Geometry check sheet. Reference: the model listing, model coordinates, mm. Face numbers are marked on the shaded views. A direction names the side the tool comes from. Give positions to 0.01 mm unless a question says otherwise; leave off trailing zeros. Loops run counter-clockwise (first coordinate to the right, second up) from the corner with the lowest first, then second, coordinate; pieces in that order, holes last. Notation, with made-up numbers: (84.25, 15) -> (143.25, 15) arc R16 ccw to (143.25, 44) -> close; hole circle Ø9 at (18.25, -29.75). An arc over 180 degrees is marked (long way). Write item = value, one per line.
```python
from build123d import *

# Parameters (mm, degrees)
ENLEV_MAT_EXTRU_1_DEPTH = 1.2
ESQUISSE3_W             = 2.5
ESQUISSE3_H             = 6
CHANFREIN1_SIZE         = 0.5
ENL_V_MAT_EXTRU_1_DEPTH = 2


with BuildPart() as part:
    # Esquisse1 → Base-R_volution (revolve)
    with BuildSketch(Plane(origin=(0, 0, 0), x_dir=(1, 0, 0), z_dir=(0, 1, 0)), mode=Mode.PRIVATE) as base_r_volution_sk:
        with BuildLine():
            Line((0, 0), (3.85, 0))
            Line((3.85, 0), (3.85, 1.47314887))
            ThreePointArc((3.85, 1.47314887), (3.806875399, 1.689977873), (3.684065354, 1.873804531))
            ThreePointArc((3.684065354, 1.873804531), (1.993841151, 3.003350962), (0, 3.4))
            Line((0, 3.4), (0, 0))
        make_face()
    revolve(base_r_volution_sk.sketch.rotate(Axis((0, 0, 0), (0, 0, -1)), 180), axis=Axis((0, 0, 0), (0, 0, -1)))

    # Esquisse2 → Enlev. mat.-Extru.1 (cut)
    with BuildSketch(Plane.XY.offset(-3.4)):
        Polygon((0.6, -0.6), (0.6, -2.35), (-0.6, -2.35), (-0.6, -0.6), (-2.35, -0.6), (-2.35, 0.6), (-0.6, 0.6), (-0.6, 2.35), (0.6, 2.35), (0.6, 0.6), (2.35, 0.6), (2.35, -0.6), align=None)
    extrude(amount=ENLEV_MAT_EXTRU_1_DEPTH, mode=Mode.SUBTRACT)

    # Esquisse3 → Boss.-R_vol.1 (revolve)
    with BuildSketch(Plane(origin=(0, 0, 0), x_dir=(1, 0, 0), z_dir=(0, 1, 0)), mode=Mode.PRIVATE) as boss_r_vol_1_sk:
        with Locations((1.25, -3)):
            Rectangle(ESQUISSE3_W, ESQUISSE3_H)
    revolve(boss_r_vol_1_sk.sketch.rotate(Axis((0, 0, 0), (0, 0, 1)), 345.677280022), axis=Axis((0, 0, 0), (0, 0, 1)))

    # Chanfrein1
    chanfrein1_edges = [part.edges().sort_by_distance(p)[0] for p in [
        (-2.422294277, 0.618458113, 6),
    ]]
    chamfer(chanfrein1_edges, length=CHANFREIN1_SIZE)

    # Esquisse6 → Enl_v. mat.-Extru.1 (cut)
    with BuildSketch(Plane(origin=(0, 0, -2.2), x_dir=(-1, 0, 0), z_dir=(0, 0, -1))):
        Polygon((2.35, -0.6), (2.35, 0.6), (0.6, 0.6), (0.6, 2.35), (-0.6, 2.35), (-0.6, 0.6), (-2.35, 0.6), (-2.35, -0.6), (-0.6, -0.6), (-0.6, -2.35), (0.6, -2.35), (0.6, -0.6), align=None)
    extrude(amount=-ENL_V_MAT_EXTRU_1_DEPTH, mode=Mode.SUBTRACT)


solid = part.part
```
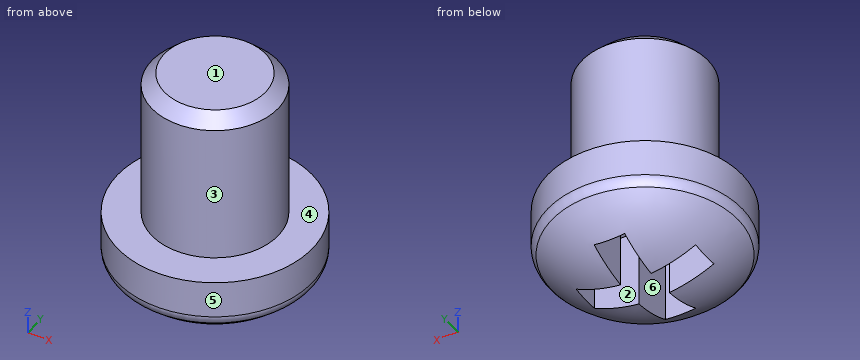
Item 1: Section check D-D, the plane z = 5. Record the cut outline in (x, y), plus the area to 3 significant figures.
Answer:
outline = circle Ø5 at (0, 0)
area = 19.6 mm^2
Item 2: Gauge pin test, flat ends, axial feed: pin 1 (1.9 mm diameter, centred on y = 1.5, z = -1, fed in from +X); pin 2 (1.4 mm diameter, centred on x = 0, y = 0.5, fed in from -Z); pin 3 (0.5 mm diameter, centred on y = 1, z = -1, fed in from -X); pin 4 (0.9 mm diameter, centred on y = -1.5, z = -2, fed in from -X). Record the tip position at first contact, or that the pin passes through.
Answer:
pin_1 = 3.81
pin_2 = -3.33
pin_3 = -3.78
pin_4 = -3.62
Item 3: Tool access check on the marked faces 4, 5 and 6. Record the directions out of +Z, -Z, +X, -X, +Y, -Y that give a thin tool (end or side, any length) a straight path to the whole face; none if there is none.
Answer:
face_4 = +Z
face_5 = +Z, -Z
face_6 = -Z
Item 4: Section check B-B, the plane x = 0. Record the cut outline in (y, z), plus the area to 3 significant figures.
Answer:
outline = (-3.85, -1.47) arc R0.57 ccw to (-3.68, -1.87) arc R5.21 ccw to (-2.35, -2.84) -> (-2.35, -0.2) -> (2.35, -0.2) -> (2.35, -2.84) arc R5.21 ccw to (3.68, -1.87) arc R0.57 ccw to (3.85, -1.47) -> (3.85, 0) -> (2.5, 0) -> (2.5, 5.5) -> (2, 6) -> (-2, 6) -> (-2.5, 5.5) -> (-2.5, 0) -> (-3.85, 0) -> close
area = 37.7 mm^2
Item 5: Thickness scan on L1, parallel to X at y = -1, z = -0.5; L2, parallel to Y at x = 0.25, z = -0.25; L3, parallel to Y at x = -2, z = -0.25. Record the ranges inside material, lowest first. Write a range as [from, to].
Answer:
L1 = [-3.72, -0.6], [0.6, 3.72]
L2 = [-3.84, -2.35], [2.35, 3.84]
L3 = [-3.29, -0.6], [0.6, 3.29]
Item 6: Section check A-A, the plane z = -0.75. Record the cut outline in (x, y), plus the area to 3 significant figures.
Answer:
outline = circle Ø7.7 at (0, 0); hole (-2.35, -0.6) -> (-0.6, -0.6) -> (-0.6, -2.35) -> (0.6, -2.35) -> (0.6, -0.6) -> (2.35, -0.6) -> (2.35, 0.6) -> (0.6, 0.6) -> (0.6, 2.35) -> (-0.6, 2.35) -> (-0.6, 0.6) -> (-2.35, 0.6) -> close
area = 36.7 mm^2
Item 7: Draft check along X on the marked faces 1, 2 and 3. Enter one of: +X half, -X half, draft (parallel to the pull), parting line (faces both ways), or undercut.
Answer:
face_1 = draft
face_2 = undercut
face_3 = parting line
